Build history of the part. All positions in model axes, mm. Face numbers are marked on the shaded views. Round coordinates to 2 decimals unless told otherwise and drop trailing zeros. Order: outer loops, then holes, each group sorted by start corner. A loop starts at its lowest first (then second) coordinate and runs counter-clockwise, first axis right, second up. Notation, with made-up numbers: (-29.75, -26) -> (18.25, -26) arc R27 ccw to (18.25, 13) -> close; hole circle Ø10 at (4.5, -0.5). An arc over 180 degrees is marked (long way). Write item = value, one per line.
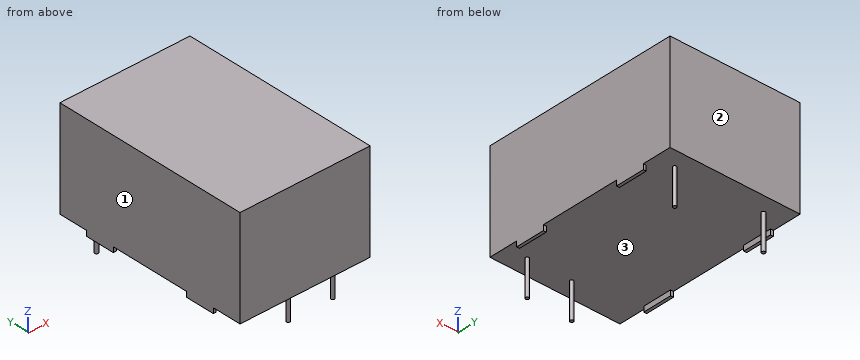
from build123d import *

# Parameters (mm, degrees)
F0_W     = 22.32
F0_H     = 33.7
F1_DEPTH = 17
F2_R     = 0.3
F3_DEPTH = 6.1
F2_W     = 0.5
F2_H     = 5
F4_DEPTH = 0.9


with BuildPart() as f1:
    # F0 (on Top) → F1 (new body)
    with BuildSketch(Plane.XY):
        Rectangle(F0_W, F0_H)
    extrude(amount=F1_DEPTH)

    # F2 (on face) → F3 (join)
    with BuildSketch(Plane(origin=(0, 0, 0), x_dir=(1, 0, 0), z_dir=(0, 0, -1))):
        with Locations((-0.11, 13.83)):
            Circle(F2_R)
        with Locations((7.51, 13.83)):
            Circle(F2_R)
        with Locations((-7.51, -13.99)):
            Circle(F2_R)
        with Locations((7.73, -13.99)):
            Circle(F2_R)
    extrude(amount=F3_DEPTH)

    # F2 (on face) → F4 (join)
    with BuildSketch(Plane(origin=(0, 0, 0), x_dir=(1, 0, 0), z_dir=(0, 0, -1))):
        with Locations((-10.91, 9.35)):
            Rectangle(F2_W, F2_H)
        with Locations((10.91, 9.35)):
            Rectangle(F2_W, F2_H)
        with Locations((-10.91, -9.35)):
            Rectangle(F2_W, F2_H)
        with Locations((10.91, -9.35)):
            Rectangle(F2_W, F2_H)
    extrude(amount=F4_DEPTH)


solid = f1.part
Q1. Cut at B-B, the plane y = 3. List the corners of the cut face in (x, z), and give its area (3 significant figures).
Check values:
outline = (-11.16, 0) -> (11.16, 0) -> (11.16, 17) -> (-11.16, 17) -> close
area = 379 mm²
Q2. Mould opens along X. For the marked faces 1, 2 and 3 say: released by +X, released by -X, zero draft, split by the parting line, or undercut.
Check values:
face_1 = released by -X
face_2 = zero draft
face_3 = undercut
Q3. Cut at A-A, the plane x = -3.25. List the corners of the cut face in (y, z).
Check values:
outline = (-16.85, 0) -> (16.85, 0) -> (16.85, 17) -> (-16.85, 17) -> close
Q4. Probe probe 1 along Z at (x, y) = (0.75, 4); probe 2 along X at (y, z) = (-14, -4.25). List the from-to ranges inside material, lowest first.
Check values:
probe_1 = 0 to 17
probe_2 = -0.36 to 0.14, 7.26 to 7.76
Q5. Flat gauge pins, fed straight in: pin 1 (12 mm diameter, centred on x = 7.5, y = 8, fed in from -Z); pin 2 (0.6 mm diameter, centred on x = -11, z = -0.5, fed in from +Y); pin 3 (0.6 mm diameter, centred on x = 11, y = 9, fed in from -Z); pin 4 (0.6 mm diameter, centred on x = -11, z = -0.5, fed in from -Y). Where does each tip first touch, or does it go through?
Check values:
pin_1 = -6.1
pin_2 = 11.85
pin_3 = -0.9
pin_4 = -11.85
